Read the model definition and answer for the solid it produces. Units are mm, in the model's axes. A direction names the side the tool comes from. Give positions to 0.01 mm unless a question says otherwise; leave off trailing zeros. Order: outer loops, then holes, each group sorted by start corner. A loop starts at its lowest first (then second) coordinate and runs counter-clockwise, first axis right, second up. Notation, with made-up numbers: (-32, -4) -> (22, -4) arc R24 cw to (22, 30) -> close; hole circle Ø2 at (19.25, -24). An arc over 180 degrees is marked (long way). One line per question, with ' | ' between items. Start each with the question number.
```python
from build123d import *

# Parameters (mm, degrees)
SM_START               = -88.265
SM_BASE_FLANGE_1_DEPTH = 176.53
FILLET_3_R             = 10
FILLET_4_R             = 10
FILLET_5_R             = 10
FILLET_6_R             = 10
FILLET_7_R             = 10


# Read off the part's stored shape, not the designer's step: 基体-法兰1
with BuildPart() as part:
    # 基体-法兰1 outline → 基体-法兰1 (new body)
    with BuildSketch(Plane(origin=(0, 0, 0), x_dir=(0, 0, -1), z_dir=(1, 0, 0)).offset(SM_START)):
        Polygon((-4.503882243, 0), (0, 0), (0, 49.038822429), (-18.519411214, 49.038822429), (-18.519411214, 63.558233643), (0, 63.558233643), (0, 112.597056072), (-4.503882243, 112.597056072), (-4.503882243, 67.558233643), (-22.519411214, 67.558233643), (-22.519411214, 45.038822429), (-4.503882243, 45.038822429), align=None)
    extrude(amount=SM_BASE_FLANGE_1_DEPTH)

    # 圆角3
    fillet_3_edges = [part.edges().sort_by_distance(p)[0] for p in [
        (0, 45.038822429, 22.519411214),
        (0, 67.558233643, 22.519411214),
    ]]
    fillet(fillet_3_edges, radius=FILLET_3_R)

    # 圆角4
    # the kernel refuses this fillet: 10 mm, written as the material it adds along each edge
    with BuildSketch(Plane(origin=(-88.265, 49.038822429, 18.519411214), x_dir=(0, 1, 0), z_dir=(1, 0, 0)), Plane(origin=(-88.265, 63.558233643, 18.519411214), x_dir=(0, 0, -1), z_dir=(1, 0, 0))) as fillet_4_piece_1:
        with BuildLine():
            CenterArc((FILLET_4_R, -FILLET_4_R), FILLET_4_R, 90, 90)
            Line((0, -FILLET_4_R), (0, 0))
            Line((0, 0), (FILLET_4_R, 0))
        make_face()
    extrude(amount=176.53)

    # 圆角5
    fillet_5_edges = [part.edges().sort_by_distance(p)[0] for p in [
        (0, 63.558233643, 0),
        (0, 49.038822429, 0),
    ]]
    fillet(fillet_5_edges, radius=FILLET_5_R)

    # 圆角6
    fillet_6_edges = [part.edges().sort_by_distance(p)[0] for p in [
        (0, 45.038822429, 4.503882243),
    ]]
    fillet(fillet_6_edges, radius=FILLET_6_R)

    # 圆角7
    fillet_7_edges = [part.edges().sort_by_distance(p)[0] for p in [
        (0, 67.558233643, 4.503882243),
    ]]
    fillet(fillet_7_edges, radius=FILLET_7_R)


solid = part.part
```
Q1. Which of the six approach directions +Z, -Z, +X, -X, +Y, -Y give full straight-line access (tool end or side, diameter ignored) to faces 1 (the cylindrical face through (-1.236, 61.365, 14.769)), 2 (the flat face through (-1, 95, 4.504)), 3 (the flat face through (-1, 0, 2))?
Q2. Find the intervals of material crossed by line 1 (Y direction, x = -78, z = 2.5); line 2 (Y direction, x = 59.5, z = 3.5); line 3 (Z direction, x = -14.5, y = 98), in increasing order.
Q3. Given P1, Ø12, axis at y = 70.5, z = 14, coming from the -X side (3 decimals); P2, Ø10, axis at x = -23, z = 15.5, coming from the -Y side; P3, Ø1, axis at x = -35.5, y = 35.5, coming from the +Z side; P4, Ø6, axis at y = 39.5, z = 10, coming from the -X side, each flat-ended and moving along its own axis, determine where each tip first touches the part or whether it passes through.
Q4. Determine the mould class of faces 4 (the flat face through (-1, 18, 4.504)), 5 (the cylindrical face through (-1.24, 51.34, 14.9)), 6 (the flat face through (-1, 112.597, 2)) for opening direction Y: pulls with the +Y half, pulls with the -Y half, needs draft (parallel to the pull), parting line crosses it, or undercut.
Q5. A cutting plane is placed at B-B, the plane z = 20.75. Determine the outline of the cut face in (x, y) (3 decimals).
Q6. A cutting plane is placed at A-A, the plane y = 95. Determine the outline of the cut face in (x, z) (3 decimals).
Geometry results:
1) face 1: -Z, +X, -X | face 2: +Z, +X, -X, +Y | face 3: +Z, -Z, +X, -X, -Y
2) line 1: 0 to 45.71, 66.89 to 112.6 | line 2: 0 to 46.69, 65.9 to 112.6 | line 3: 0 to 4.5
3) P1: x = -88.265 | P2: y = 44.3 | P3: z = 4.54 | P4: through
4) face 4: needs draft | face 5: undercut | face 6: pulls with the +Y half
5) outline: (-88.265, 49.359) -> (88.265, 49.359) -> (88.265, 63.238) -> (-88.265, 63.238) -> close
6) outline: (-88.265, 0) -> (88.265, 0) -> (88.265, 4.504) -> (-88.265, 4.504) -> close
